Geometry: final body of the model. Coordinates: model frame, mm. Face numbers are marked on the shaded views. A direction names the side the tool comes from. Coordinates: 2 decimals unless noted, no trailing zeros. Write each loop counter-clockwise with the first axis right and the second up, starting at its lowest first coordinate (ties: lowest second). Pieces come first, ordered by that corner, then holes.
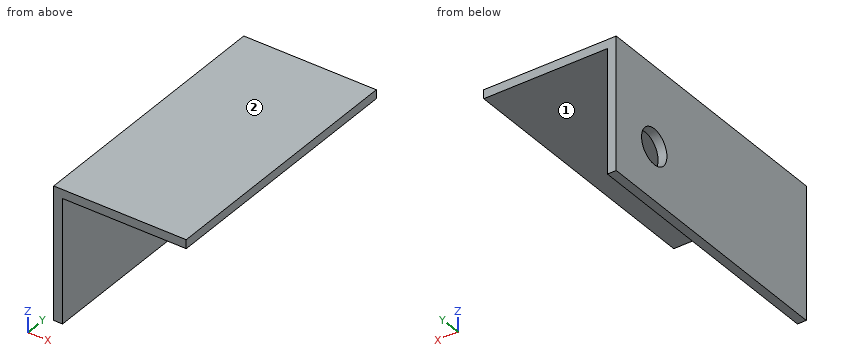
from build123d import *

# Parameters (mm, degrees)
EXTRUDE_1_DEPTH     = 150
SKETCH_2_R          = 10
CUT_EXTRUDE_1_DEPTH = 76


with BuildPart() as part:
    # Эскиз1 → Вытянуть-Тонкостенный1 (new body)
    with BuildSketch(Plane(origin=(0, 0, 0), x_dir=(1, 0, 0), z_dir=(0, 1, 0))):
        Polygon((0, 75), (0, 0), (75, 0), (75, 5), (5, 5), (5, 75), align=None)
    extrude(amount=EXTRUDE_1_DEPTH)

    # Эскиз2 → Вырез-Вытянуть1 (cut, through all)
    with BuildSketch(Plane.ZY):
        with Locations((-45, 120)):
            Circle(SKETCH_2_R)
    extrude(amount=-CUT_EXTRUDE_1_DEPTH, mode=Mode.SUBTRACT)


solid = part.part
Item 1: Section D-D, the plane y = 33. Output: boundary loops of the cut face in (x, z).
Derived:
outline: (0, -75) - (5, -75) - (5, -5) - (75, -5) - (75, 0) - (0, 0) - close
Item 2: Material intervals for probe 1 along Y at (x, z) = (2, -45); probe 2 along Z at (x, y) = (34.5, 83.5); probe 3 along X at (y, z) = (64.5, -18), sorted ascending.
Derived:
probe 1: y = 0 to 110, 130 to 150
probe 2: z = -5 to 0
probe 3: x = 0 to 5
Item 3: Pin query (flat end, axial travel): pin 1 (5 mm diameter, centred on y = 122, z = -52.5, fed in from +X). Return the tip coordinate at first contact, or that it passes through.
Derived:
pin 1: stops at x = 5
Item 4: Section C-C, the plane z = -45. Output: boundary loops of the cut face in (x, y), plus the area to 3 significant figures.
Derived:
outline: (0, 0) - (5, 0) - (5, 110) - (0, 110) - close; (0, 130) - (5, 130) - (5, 150) - (0, 150) - close
area: 650 mm2
Item 5: Set-up query: the marked faces 1 and 2. Return all of +Z, -Z, +X, -X, +Y, -Y with unobstructed straight access to the full face (end or side cutting, diameter ignored); none if empty.
Derived:
face 1: -Z, +X, +Y, -Y
face 2: +Z, +X, -X, +Y, -Y
Item 6: Section A-A, the plane z = -37. Output: boundary loops of the cut face in (x, y).
Derived:
outline: (0, 0) - (5, 0) - (5, 114) - (0, 114) - close; (0, 126) - (5, 126) - (5, 150) - (0, 150) - close
Item 7: Section B-B, the plane y = 120. Output: boundary loops of the cut face in (x, z), plus the area to 3 significant figures.
Derived:
outline: (0, -75) - (5, -75) - (5, -55) - (0, -55) - close; (0, -35) - (5, -35) - (5, -5) - (75, -5) - (75, 0) - (0, 0) - close
area: 625 mm2
